```python
from build123d import *

# Parameters (mm, degrees)
SKETCH_2_R          = 28.5
SKETCH_2_R_2        = 7.7
SKETCH_2_R_3        = 1.65
EXTRUDE_2_DEPTH     = 20
EXTRUDE_START       = -6
EXTRUDE_3_DEPTH     = 6
EXTRUDE_4_DEPTH     = 8
EXTRUDE_START_2     = 6
EXTRUDE_5_DEPTH     = 6
SKETCH_7_R          = 3
CUT_EXTRUDE_4_DEPTH = 20


# Read off the part's stored shape, not the designer's step: the extrude step
with BuildPart() as part:
    # Sketch 2 → Extrude 2 (new body)
    with BuildSketch(Plane(origin=(0, 10, 0), x_dir=(0, 0, -1), z_dir=(0, 1, 0))):
        with Locations(Location((-10.824457271, 40.125190792, 0), (0, 0, 180))):
            Circle(SKETCH_2_R)
        with Locations(Location((-10.824457271, 40.125190792, 0), (0, 0, 180))):
            Circle(SKETCH_2_R_2, mode=Mode.SUBTRACT)
        with Locations(Location((-14.303615873, 23.229689751, 0), (0, 0, 180))):
            Circle(SKETCH_2_R_3, mode=Mode.SUBTRACT)
        with Locations(Location((-27.195969683, 34.690480004, 0), (0, 0, 180))):
            Circle(SKETCH_2_R_3, mode=Mode.SUBTRACT)
        with Locations(Location((2.067896539, 28.664400538, 0), (0, 0, 180))):
            Circle(SKETCH_2_R_3, mode=Mode.SUBTRACT)
        with Locations(Location((5.547055141, 45.559901579, 0), (0, 0, 180))):
            Circle(SKETCH_2_R_3, mode=Mode.SUBTRACT)
        with Locations(Location((-7.345298669, 57.020691832, 0), (0, 0, 180))):
            Circle(SKETCH_2_R_3, mode=Mode.SUBTRACT)
        with Locations(Location((-23.716811081, 51.585981045, 0), (0, 0, 180))):
            Circle(SKETCH_2_R_3, mode=Mode.SUBTRACT)
    extrude(amount=EXTRUDE_2_DEPTH)

    # Sketch 3 → Extrude 3 (add)
    with BuildSketch(Plane(origin=(0, 30, 0), x_dir=(1, 0, 0), z_dir=(0, 1, 0)).offset(EXTRUDE_START)):
        with BuildLine():
            ThreePointArc((-25.125190792, -35.057698903), (-40.125190792, -39.324457271), (-55.125190792, -35.057698903))
            Line((-55.125190792, -35.057698903), (-55.125190792, -98.824457271))
            ThreePointArc((-55.125190792, -98.824457271), (-40.125190792, -113.824457271), (-25.125190792, -98.824457271))
            Line((-25.125190792, -98.824457271), (-25.125190792, -35.057698903))
        make_face()
    extrude(amount=EXTRUDE_3_DEPTH)

    # Extrude 4 outline → Extrude 4 (add)
    with BuildSketch(Plane(origin=(0, 24, 0), x_dir=(-1, 0, 0), z_dir=(0, -1, 0))):
        with BuildLine():
            Line((55.125190792, -68.824205807), (55.125190792, -35.057698903))
            ThreePointArc((55.125190792, -35.057698903), (40.125190792, -39.324457271), (25.125190792, -35.057698903))
            Line((25.125190792, -35.057698903), (25.125190792, -68.824205807))
            ThreePointArc((25.125190792, -68.824205807), (40.125190792, -83.824205807), (55.125190792, -68.824205807))
        make_face()
    extrude(amount=EXTRUDE_4_DEPTH)

    # Sketch 6 → Extrude 5 (add)
    with BuildSketch(Plane(origin=(0, 16, 0), x_dir=(-1, 0, 0), z_dir=(0, -1, 0)).offset(EXTRUDE_START_2)):
        with BuildLine():
            ThreePointArc((25.125190792, -98.824457271), (40.125190792, -113.824457271), (55.125190792, -98.824457271))
            Line((55.125190792, -98.824457271), (25.125190792, -98.824457271))
        make_face()
        with BuildLine():
            Line((25.125190792, -98.824457271), (55.125190792, -98.824457271))
            ThreePointArc((55.125190792, -98.824457271), (40.125190792, -83.824457271), (25.125190792, -98.824457271))
        make_face()
        with BuildLine():
            Line((55.125190792, -98.824457271), (55.125190792, -68.824205807))
            ThreePointArc((55.125190792, -68.824205807), (40.125190792, -83.824205807), (25.125190792, -68.824205807))
            Line((25.125190792, -68.824205807), (25.125190792, -98.824457271))
            ThreePointArc((25.125190792, -98.824457271), (40.125190792, -83.824457271), (55.125190792, -98.824457271))
        make_face()
        with BuildLine():
            ThreePointArc((55.125190792, -35.057698903), (40.125190792, -39.324457271), (25.125190792, -35.057698903))
            Line((25.125190792, -35.057698903), (25.125190792, -68.824205807))
            ThreePointArc((25.125190792, -68.824205807), (40.125190792, -83.824205807), (55.125190792, -68.824205807))
            Line((55.125190792, -68.824205807), (55.125190792, -35.057698903))
        make_face()
    extrude(amount=-EXTRUDE_5_DEPTH)

    # Sketch 7 → Cut-Extrude 4 (cut)
    with BuildSketch(Plane(origin=(0, 10, 0), x_dir=(-1, 0, 0), z_dir=(0, -1, 0))):
        with Locations(Location((40.125725395, -98.822710565, 0), (0, 0, 90))):
            Circle(SKETCH_7_R)
    extrude(amount=-CUT_EXTRUDE_4_DEPTH, mode=Mode.SUBTRACT)


solid = part.part
```
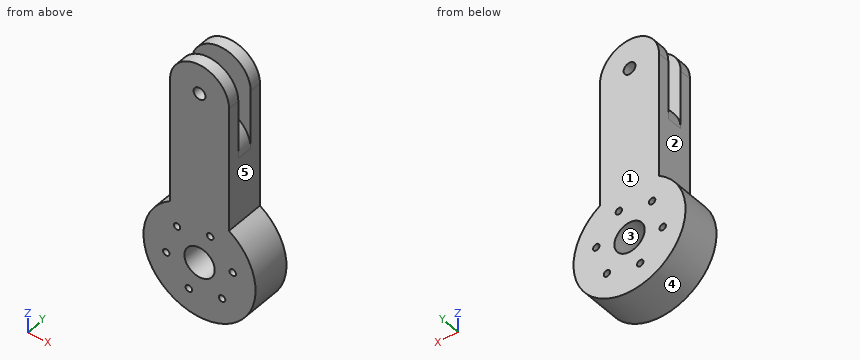
Build history of the part. All positions in model axes, mm. Face numbers are marked on the shaded views. A direction names the side the tool comes from. Round coordinates to 2 decimals unless told otherwise and drop trailing zeros. Order: outer loops, then holes, each group sorted by start corner. A loop starts at its lowest first (then second) coordinate and runs counter-clockwise, first axis right, second up. Notation, with made-up numbers: (-18, 39.5) -> (-3, 39.5) arc R18 cw to (-3, 64.5) -> close; hole circle Ø6 at (46, 29.5). An arc over 180 degrees is marked (long way). Answer in a Markdown table with one row per item.
1) Which spindle directions (+Z, -Z, +X, -X, +Y, -Y) get a long thin tool onto all of the face, cutting with end or side? Do the marked faces 4 and 5. Say none if no direction does.
Values:
| item | result |
|---|---|
| face 4 | +Y, -Y |
| face 5 | +Z, +X, +Y, -Y |
2) Pin check, flat tips, straight feed: P1, Ø9.5, axis at x = -40.13, z = 98.82, coming from the -Y side; P2, Ø6, axis at x = -25.5, y = 13, coming from the -Z side; P3, Ø6, axis at y = 20, z = 59.5, coming from the +X side; P4, Ø4, axis at x = -35, y = 14, coming from the +Z side. Stop position of each tip, or through.
Values:
| item | result |
|---|---|
| P1 | y = 10 |
| P2 | z = -15.2 |
| P3 | x = -25.13 |
| P4 | z = 113.5 |
3) Band-saw the part on B-B on y = 12.5. Give the number of separate pieces and of enclosed holes in the cut face, and give its area (3 significant figures).
Values:
| item | result |
|---|---|
| separate pieces | 1 |
| enclosed holes | 8 |
| area | 4,470 mm2 |
4) Mould opens along X. For the marked faces 1, 2 and 3 say: released by +X, released by -X, zero draft, split by the parting line, or undercut.
Values:
| item | result |
|---|---|
| face 1 | zero draft |
| face 2 | released by -X |
| face 3 | undercut |
5) Band-saw the part on C-C on y = 21.75. Give the cut face in (x, z), and give its area (3 significant figures).
Values:
| item | result |
|---|---|
| outline | (-55.13, 35.06) arc R28.5 ccw (long way) to (-25.13, 35.06) -> (-25.13, 68.82) arc R15 ccw to (-55.13, 68.82) -> close; hole circle Ø3.3 at (-57.02, 7.35); hole circle Ø3.3 at (-51.59, 23.72); hole circle Ø15.4 at (-40.13, 10.82); hole circle Ø3.3 at (-45.56, -5.55); hole circle Ø3.3 at (-34.69, 27.2); hole circle Ø3.3 at (-28.66, -2.07); hole circle Ø3.3 at (-23.23, 14.3) |
| area | 3,590 mm2 |
6) Band-saw the part on A-A on z = 91. Give the cut face in (x, y).
Values:
| item | result |
|---|---|
| outline | (-55.13, 10) -> (-25.13, 10) -> (-25.13, 16) -> (-55.13, 16) -> close; (-55.13, 24) -> (-25.13, 24) -> (-25.13, 30) -> (-55.13, 30) -> close |
7) Wall check: L1, parallel to Z at x = -35, y = 21.5; L2, parallel to Z at x = -45, y = 18.75; L3, parallel to Y at x = -40, z = 108. Give the ranges that are in metal, low to high.
Values:
| item | result |
|---|---|
| L1 | -17.21 to 5.08, 16.57 to 25.58, 28.82 to 82.92 |
| L2 | -17.26 to -7.1, -3.99 to 4.86, 16.78 to 83.01 |
| L3 | 10 to 16, 24 to 30 |
8) Band-saw the part on D-D on z = 76.5. Give the cut face in (x, y), and give its area (3 significant figures).
Values:
| item | result |
|---|---|
| outline | (-55.13, 10) -> (-25.13, 10) -> (-25.13, 16) -> (-27.24, 16) -> (-27.24, 24) -> (-25.13, 24) -> (-25.13, 30) -> (-55.13, 30) -> (-55.13, 24) -> (-53.01, 24) -> (-53.01, 16) -> (-55.13, 16) -> close |
| area | 566 mm2 |
